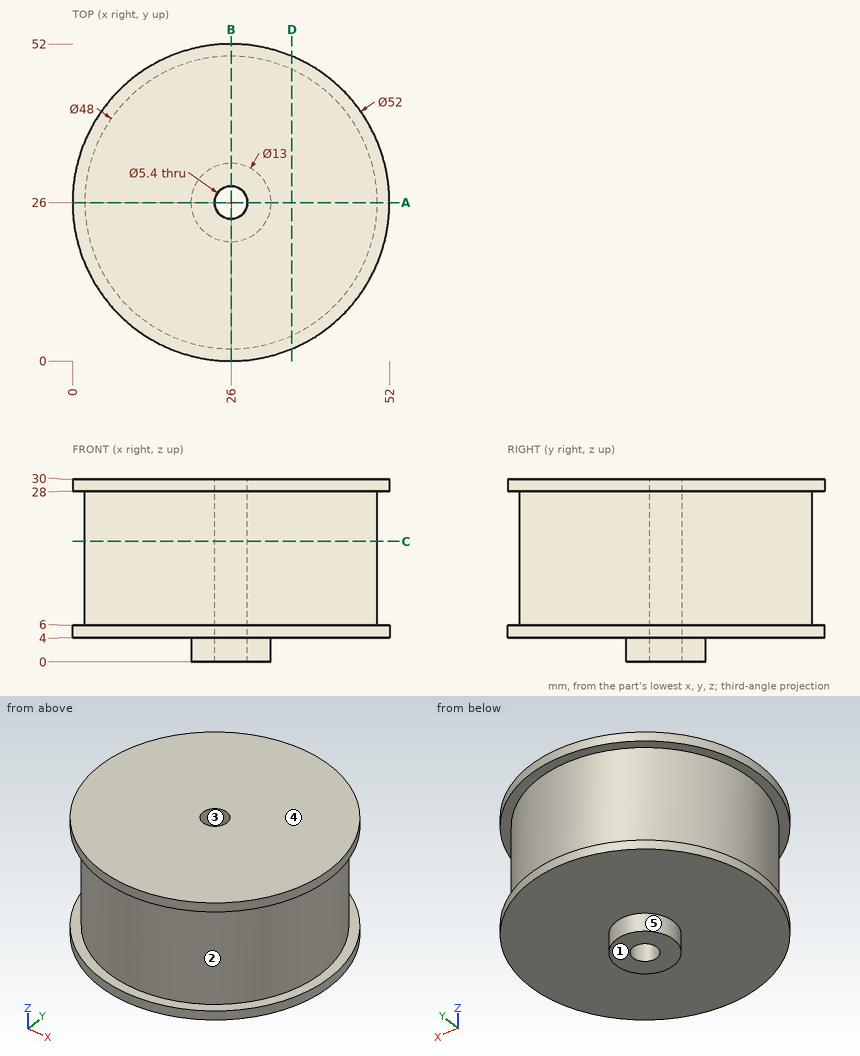
Answer from the drawing. Dimensions are ordinates in mm from the lowest x, y and z of the part. A direction names the side the tool comes from. Coordinates: 2 decimals unless noted, no trailing zeros. Loops run counter-clockwise (first coordinate to the right, second up) from the corner with the lowest first, then second, coordinate; pieces in that order, holes last.
Q1. Consider probe 1 along Z at (x, y) = (4.5, 13.5); probe 2 along Y at (x, z) = (26, 16.25); probe 3 along X at (y, z) = (28, 13.25). Determine where each line is inside the solid, lowest interval first.
Q2. Which of the six approach directions +Z, -Z, +X, -X, +Y, -Y give full straight-line access (tool end or side, diameter ignored) to the marked faces 4 and 5?
Q3. The part is cut by section D-D on x = 36. Write down the section's boundary in (y, z), and give its area (3 significant figures).
Q4. The part is cut by section A-A on y = 26. Write down the section's boundary in (x, z), and give its area (3 significant figures).
Q5. Each of these flat-tipped pins is pushed along its axis until it touches: pin 1 Ø10 at (x, y) = (38.5, 40.5) entering from -Z; pin 2 Ø4 at (y, z) = (24.5, 22) entering from -X; pin 3 Ø7 at (x, y) = (26, 26) entering from +Z; pin 4 Ø1.5 at (y, z) = (23.5, 8.5) entering from -X. Where does it stop, or does it pass through?
Q6. The part is cut by section C-C on z = 19.75. Write down the section's boundary in (x, y), and give its area (3 significant figures).
Q7. The mould has two halves that part along X. Classify the marked faces 1, 2 and 3: +X half, -X half, draft (parallel to the pull), parting line (faces both ways), or undercut.
Results below:
1. probe 1: z = 4 to 6, 28 to 30
1. probe 2: y = 2 to 23.3, 28.7 to 50
1. probe 3: x = 2.08 to 24.19, 27.81 to 49.92
2. face 4: +Z, +X, -X, +Y, -Y
2. face 5: -Z
3. outline: (2, 4) - (50, 4) - (50, 6) - (47.82, 6) - (47.82, 28) - (50, 28) - (50, 30) - (2, 30) - (2, 28) - (4.18, 28) - (4.18, 6) - (2, 6) - close
3. area: 1,150 mm2
4. outline: (0, 4) - (19.5, 4) - (19.5, 0) - (23.3, 0) - (23.3, 30) - (0, 30) - (0, 28) - (2, 28) - (2, 6) - (0, 6) - close; (28.7, 0) - (32.5, 0) - (32.5, 4) - (52, 4) - (52, 6) - (50, 6) - (50, 28) - (52, 28) - (52, 30) - (28.7, 30) - close
4. area: 1,150 mm2
5. pin 1: stops at z = 4
5. pin 2: stops at x = 2
5. pin 3: stops at z = 30
5. pin 4: stops at x = 2.06
6. outline: circle Ø48 at (26, 26); hole circle Ø5.4 at (26, 26)
6. area: 1,790 mm2
7. face 1: draft
7. face 2: parting line
7. face 3: undercut
